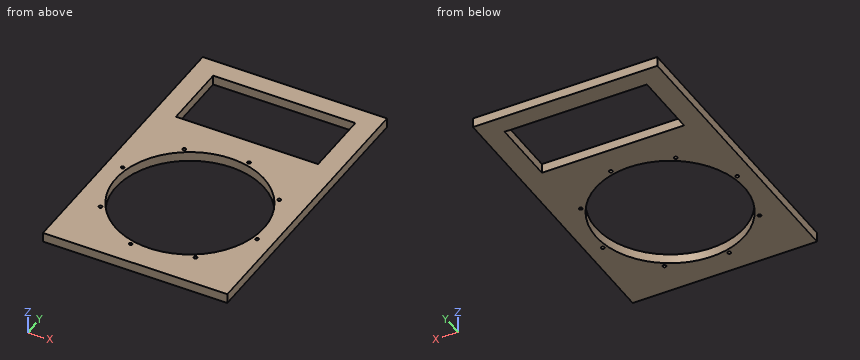
from build123d import *

# Parameters (mm, degrees)
SKETCH1_W           = 345.7
SKETCH1_H           = 544.6
BOSS_EXTRUDE1_DEPTH = 18
SKETCH2_W           = 266.7
SKETCH2_H           = 127
CUT_EXTRUDE1_DEPTH  = 19
SKETCH3_R           = 139.065
CUT_EXTRUDE2_DEPTH  = 19
SKETCH4_R           = 3.175
CUT_EXTRUDE3_DEPTH  = 19


with BuildPart() as part:
    # Sketch1 → Boss-Extrude1 (new body)
    with BuildSketch(Plane.XY):
        with Locations((172.85, 272.3)):
            Rectangle(SKETCH1_W, SKETCH1_H)
    extrude(amount=BOSS_EXTRUDE1_DEPTH)

    # Sketch2 → Cut-Extrude1 (cut, through all)
    with BuildSketch(Plane.XY.offset(18)):
        with Locations((172.85, 445)):
            Rectangle(SKETCH2_W, SKETCH2_H)
    extrude(amount=-CUT_EXTRUDE1_DEPTH, mode=Mode.SUBTRACT)

    # Sketch3 → Cut-Extrude2 (cut, through all)
    with BuildSketch(Plane.XY.offset(18)):
        with Locations((172.85, 186.690965799)):
            Circle(SKETCH3_R)
    extrude(amount=-CUT_EXTRUDE2_DEPTH, mode=Mode.SUBTRACT)

    # Sketch4 → Cut-Extrude3 (cut, through all)
    with BuildSketch(Plane.XY.offset(18)):
        with Locations((204.842157428, 330.365184475)):
            Circle(SKETCH4_R)
        with Locations((297.06488577, 265.662108644)):
            Circle(SKETCH4_R)
        with Locations((316.524218676, 154.698808371)):
            Circle(SKETCH4_R)
        with Locations((251.821142845, 62.476080029)):
            Circle(SKETCH4_R)
        with Locations((140.857842572, 43.016747123)):
            Circle(SKETCH4_R)
        with Locations((48.63511423, 107.719822954)):
            Circle(SKETCH4_R)
        with Locations((29.175781324, 218.683123227)):
            Circle(SKETCH4_R)
        with Locations((93.878857155, 310.905851569)):
            Circle(SKETCH4_R)
    extrude(amount=-CUT_EXTRUDE3_DEPTH, mode=Mode.SUBTRACT)


solid = part.part
Verification items for the finished model (mm, model axes). Coordinates: 2 decimals unless noted, no trailing zeros. Write each loop counter-clockwise with the first axis right and the second up, starting at its lowest first coordinate (ties: lowest second). Pieces come first, ordered by that corner, then holes. Notation, with made-up numbers: (-39.5, 76.5) - (-15.5, 76.5) arc R24 cw to (-15.5, 110.5) - close; hole circle Ø9 at (74.5, 82.5). An arc over 180 degrees is marked (long way). Answer as a JSON object with one key per item and string values.
(1) Cross-section at C-C on z = 15. Give the number of separate pieces and of enclosed holes in the cut face, plus the area to 3 significant figures.
Report:
{"separate pieces": "1", "enclosed holes": "10", "area": "93,400 mm^2"}
(2) Cross-section at D-D on x = 240. Record the cut outline in (y, z).
Report:
{"outline": "(0, 0) - (64.91, 0) - (64.91, 18) - (0, 18) - close; (308.47, 0) - (381.5, 0) - (381.5, 18) - (308.47, 18) - close; (508.5, 0) - (544.6, 0) - (544.6, 18) - (508.5, 18) - close"}
(3) Thickness scan on line 1 along Y through (x, z) = (172, 6.5); line 2 along Y through (x, z) = (178.5, 8.75); line 3 along X through (y, z) = (496.5, 6.5). Record the ranges inside material, lowest first.
Report:
{"line 1": "0 to 47.63, 325.75 to 381.5, 508.5 to 544.6", "line 2": "0 to 47.74, 325.64 to 381.5, 508.5 to 544.6", "line 3": "0 to 39.5, 306.2 to 345.7"}
(4) Cross-section at A-A on x = 172.85. Record the cut outline in (y, z).
Report:
{"outline": "(0, 0) - (47.63, 0) - (47.63, 18) - (0, 18) - close; (325.76, 0) - (381.5, 0) - (381.5, 18) - (325.76, 18) - close; (508.5, 0) - (544.6, 0) - (544.6, 18) - (508.5, 18) - close"}
(5) Cross-section at B-B on y = 438. Record the cut outline in (x, z).
Report:
{"outline": "(0, 0) - (39.5, 0) - (39.5, 18) - (0, 18) - close; (306.2, 0) - (345.7, 0) - (345.7, 18) - (306.2, 18) - close"}
